Drawing for the job (mm, zero at the part's lowest x, y, z). A direction names the side the tool comes from. Give positions to 0.01 mm unless a question says otherwise; leave off trailing zeros. Loops run counter-clockwise (first coordinate to the right, second up) from the corner with the lowest first, then second, coordinate; pieces in that order, holes last. Notation, with made-up numbers: (-35.75, -28.5) -> (-3.75, -28.5) arc R16 ccw to (-3.75, -19.5) -> close; hole circle Ø10 at (-5, 71.5). An arc over 180 degrees is marked (long way). Answer in a Markdown table with one row per item. Add a question column.
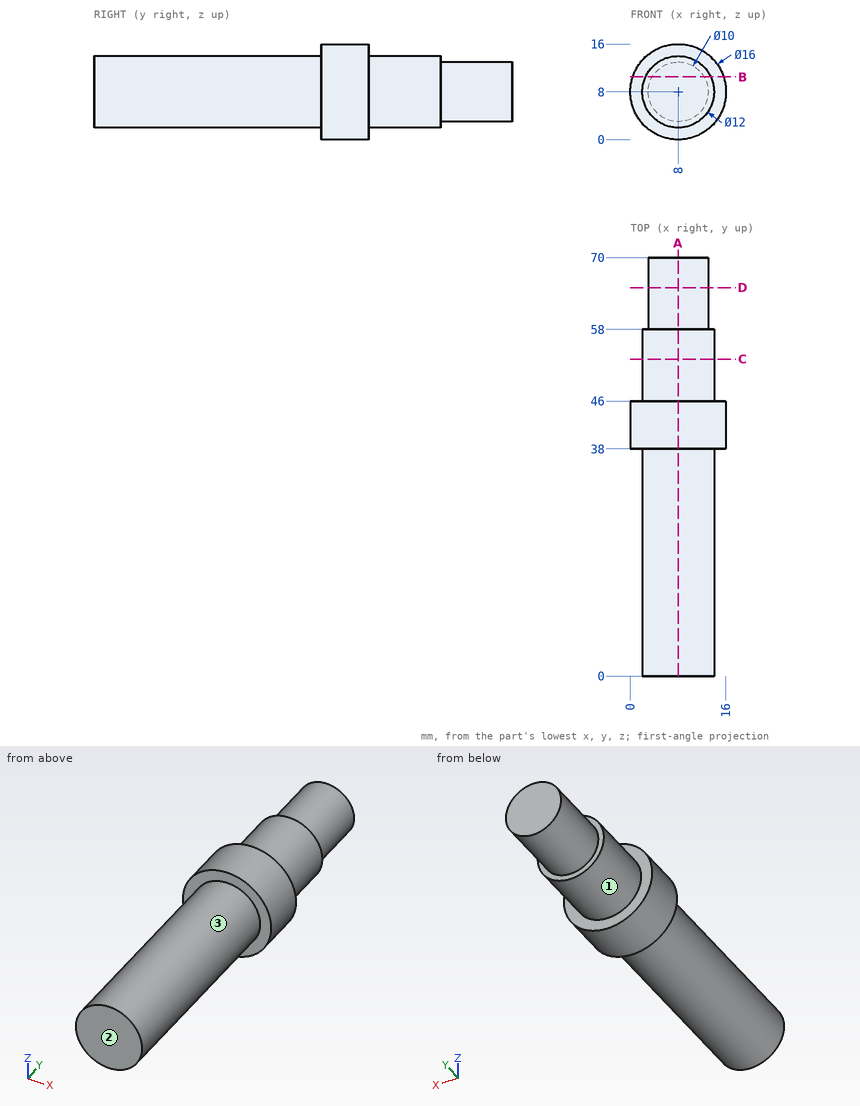
(1) 3-axis set-ups, long thin cutter, end or side, ignore diameter. For the marked faces 1, 2 and 3: which of +Z, -Z, +X, -X, +Y, -Y reach the whole face in a straight line?
(2) Saw through at B-B, the plane z = 10.5. List the corners of the cut face in (x, y).
(3) Saw through at D-D, the plane y = 65. List the corners of the cut face in (x, z), then the cut area to 3 significant figures.
(4) Wall check: line 1 along Y through (x, z) = (2.5, 11.75); line 2 along X through (y, z) = (19.5, 11.5); line 3 along Z through (x, y) = (8.5, 34). Give the ranges that are in metal, low to high. Write a range as from..to.
(5) Flat gauge pins, fed straight in: pin 1 Ø5 at (x, y) = (6.5, 30) entering from +Z; pin 2 Ø1.5 at (y, z) = (44.5, 12.5) entering from -X; pin 3 Ø2 at (x, y) = (8, 60) entering from +Z. Where does each tip first touch, or does it go through?
(6) Saw through at C-C, the plane y = 53. List the corners of the cut face in (x, z), then the cut area to 3 significant figures.
(7) Saw through at A-A, the plane x = 8. List the corners of the cut face in (y, z), then the cut area to 3 significant figures.
Worked answers:
| question | item | result |
|---|---|---|
| 1 | face 1 | +Y |
| 1 | face 2 | +Z, -Z, +X, -X, -Y |
| 1 | face 3 | -Y |
| 2 | outline | (0.4, 38) -> (2.55, 38) -> (2.55, 0) -> (13.45, 0) -> (13.45, 38) -> (15.6, 38) -> (15.6, 46) -> (13.45, 46) -> (13.45, 58) -> (12.33, 58) -> (12.33, 70) -> (3.67, 70) -> (3.67, 58) -> (2.55, 58) -> (2.55, 46) -> (0.4, 46) -> close |
| 3 | outline | circle Ø10 at (8, 8) |
| 3 | area | 78.5 mm^2 |
| 4 | line 1 | 38..46 |
| 4 | line 2 | 3.13..12.87 |
| 4 | line 3 | 2.02..13.98 |
| 5 | pin 1 | z = 14 |
| 5 | pin 2 | x = 0.93 |
| 5 | pin 3 | z = 13 |
| 6 | outline | circle Ø12 at (8, 8) |
| 6 | area | 113 mm^2 |
| 7 | outline | (0, 2) -> (38, 2) -> (38, 0) -> (46, 0) -> (46, 2) -> (58, 2) -> (58, 3) -> (70, 3) -> (70, 13) -> (58, 13) -> (58, 14) -> (46, 14) -> (46, 16) -> (38, 16) -> (38, 14) -> (0, 14) -> close |
| 7 | area | 848 mm^2 |
